```python
from build123d import *

# Parameters (mm, degrees)
BOSS_EXTRUDE1_DEPTH = 15


with BuildPart() as part:
    # Sketch1 → Boss-Extrude1 (new body)
    with BuildSketch(Plane(origin=(0, 0, 0), x_dir=(1, 0, 0), z_dir=(0, 1, 0))):
        with BuildLine():
            ThreePointArc((8.85981646, -36.734366282), (51.162558776, 11.169517142), (-12.744491466, 10.7302178))
            Line((-12.744491466, 10.7302178), (-25.946747838, -19.365677712))
            ThreePointArc((-25.946747838, -19.365677712), (-28.156287224, -21.87397008), (-31.410106737, -22.639641991))
            Line((-31.410106737, -22.639641991), (-42.677134679, -21.762954271))
            ThreePointArc((-42.677134679, -21.762954271), (-52.722336819, -36.115449465), (-35.30183314, -37.966464293))
            Line((-35.30183314, -37.966464293), (-28.563233928, -28.894210954))
            ThreePointArc((-28.563233928, -28.894210954), (-25.848867686, -26.943362215), (-22.506228219, -26.924486508))
            Line((-22.506228219, -26.924486508), (8.85981646, -36.734366282))
        make_face()
        with BuildLine():
            Line((-42.754710221, -22.759940748), (-31.487682279, -23.636628468))
            ThreePointArc((-31.487682279, -23.636628468), (-27.642259218, -22.731743482), (-25.030985399, -19.767397956))
            Line((-25.030985399, -19.767397956), (-11.828729026, 10.328497556))
            ThreePointArc((-11.828729026, 10.328497556), (50.252405495, 10.755245488), (9.158312959, -35.779955553))
            Line((9.158312959, -35.779955553), (-22.20773172, -25.970075778))
            ThreePointArc((-22.20773172, -25.970075778), (-26.158123817, -25.992383432), (-29.366011194, -28.297931942))
            Line((-29.366011194, -28.297931942), (-36.104610407, -37.370185281))
            ThreePointArc((-36.104610407, -37.370185281), (-51.812183538, -35.701177811), (-42.754710221, -22.759940748))
        make_face(mode=Mode.SUBTRACT)
    extrude(amount=BOSS_EXTRUDE1_DEPTH)


solid = part.part
```
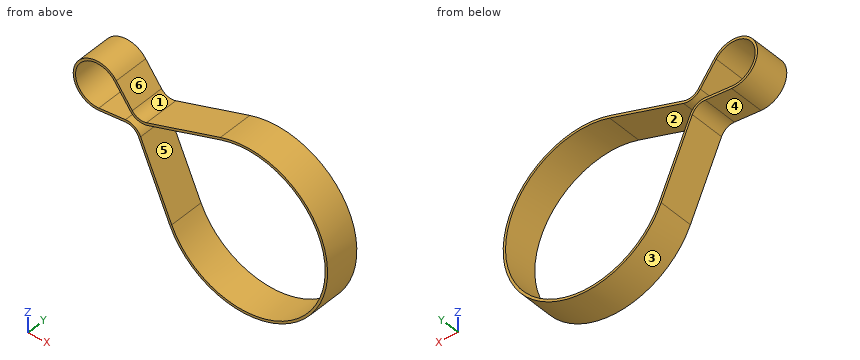
Check sheet for the modelled part. Datum: model origin and axes. Units: mm. Face numbers are marked on the shaded views. A direction names the side the tool comes from. Coordinates: 2 decimals unless noted, no trailing zeros. Loops run counter-clockwise (first coordinate to the right, second up) from the corner with the lowest first, then second, coordinate; pieces in that order, holes last.
1) Sectioned sample at B-B (x = 0). Record the boundary of the cut face in (y, z).
2) Release check for a two-part mould opening along Z. For the marked faces 1, 2 and 3 record: released by +Z, released by -Z, zero draft, split by the parting line, or undercut.
3) Sectioned sample at A-A (z = -12.5). Record the boundary of the cut face in (x, y).
4) Sectioned sample at C-C (y = 7.25). Record the boundary of the cut face in (x, z).
5) Access from +Z, -Z, +X, -X, +Y, -Y to the whole of each face (thin tool, end or side, straight path). Record for the marked faces 4, 5 and 6.
6) Material ranges on probe 1 along X at (y, z) = (11.5, 6); probe 2 along Z at (x, y) = (-47, 3.5); probe 3 along Z at (x, y) = (5, 7.25), recorded low to high.
7) Gauge pin test, flat ends, axial feed: pin 1 (1 mm diameter, centred on x = 18.5, y = 2, fed in from +Z); pin 2 (8 mm diameter, centred on y = 4.5, z = 5, fed in from -X); pin 3 (6 mm diameter, centred on y = 11.5, z = 28, fed in from +X). Record the tip position at first contact, or that the pin passes through.
Check sheet entries:
1. outline: (0, -25.86) - (15, -25.86) - (15, -24.66) - (0, -24.66) - close; (0, 32.92) - (15, 32.92) - (15, 33.96) - (0, 33.96) - close
2. face 1: released by +Z
2. face 2: undercut
2. face 3: split by the parting line
3. outline: (-11.91, 0) - (-10.78, 0) - (-10.78, 15) - (-11.91, 15) - close; (49.4, 0) - (50.52, 0) - (50.52, 15) - (49.4, 15) - close
4. outline: (-42.68, 21.76) - (-31.41, 22.64) arc R5.5 cw to (-25.95, 19.37) - (-12.74, -10.73) arc R35 ccw (long way) to (8.86, 36.73) - (-22.51, 26.92) arc R5.5 cw to (-28.56, 28.89) - (-35.3, 37.97) arc R10.17 ccw (long way) to start; hole (-42.75, 22.76) - (-31.49, 23.64) arc R6.5 cw to (-25.03, 19.77) - (-11.83, -10.33) arc R34 ccw (long way) to (9.16, 35.78) - (-22.21, 25.97) arc R6.5 cw to (-29.37, 28.3) - (-36.1, 37.37) arc R9.17 ccw (long way) to start
5. face 4: -Z, +Y, -Y
5. face 5: +Y, -Y
5. face 6: +Z, +Y, -Y
6. probe 1: x = -20.08 to -18.99, 53.2 to 54.21
6. probe 2: z = 22.37 to 23.44, 40.36 to 41.44
6. probe 3: z = -28.61 to -27.51, 34.48 to 35.53
7. pin 1: stops at z = 38.33
7. pin 2: stops at x = -21.4
7. pin 3: stops at x = 46.79
